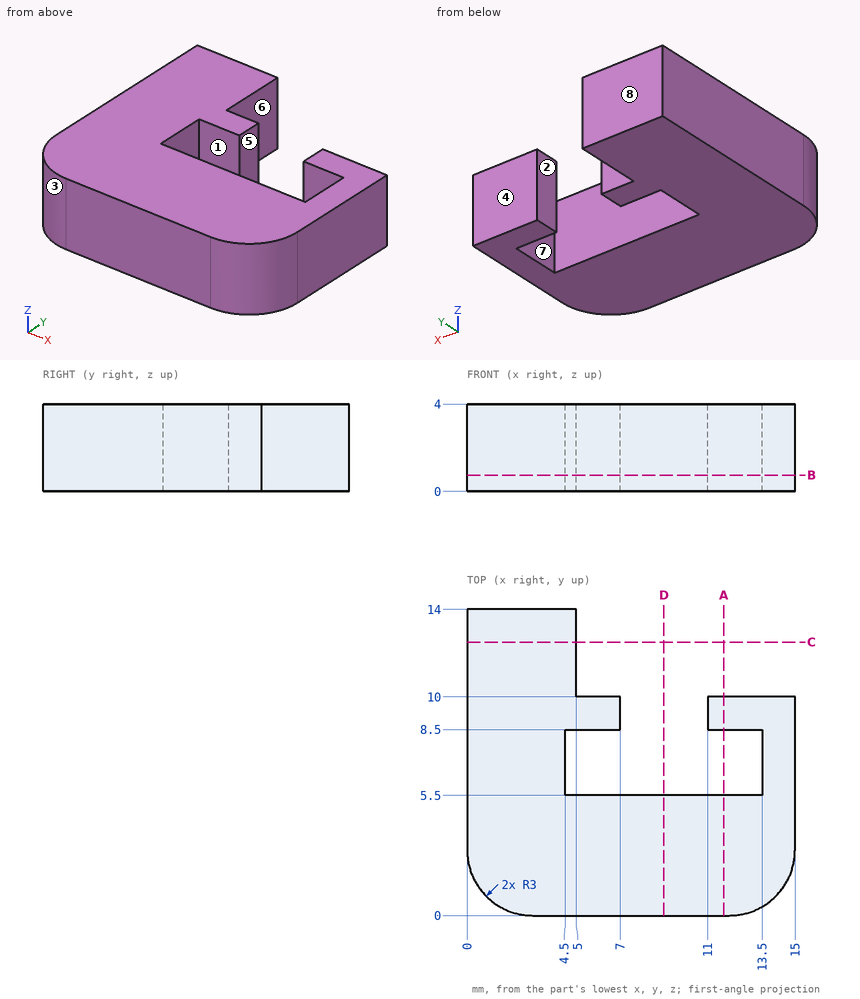
For this review, use the dimensioned drawing (mm, ordinates from the lowest corner) and the shaded views. A direction names the side the tool comes from. Give positions to 0.01 mm unless a question says otherwise; leave off trailing zeros. Order: outer loops, then holes, each group sorted by start corner. A loop starts at its lowest first (then second) coordinate and runs counter-clockwise, first axis right, second up.
1. Add section A-A, the plane x = 11.75. State the section outline as (y, z) points.
Solution:
outline: (0, 0) - (5.5, 0) - (5.5, 4) - (0, 4) - close; (8.5, 0) - (10, 0) - (10, 4) - (8.5, 4) - close
2. To check wall thickness, follow L1, parallel to X at y = 9.5, z = 0.5; L2, parallel to Y at x = 6, z = 2.2; L3, parallel to X at y = 7, z = 2.3. State the ranges of each line that lie inside material, in increasing order.
Solution:
L1: x = 0 to 7, 11 to 15
L2: y = 0 to 5.5, 8.5 to 10
L3: x = 0 to 4.5, 13.5 to 15
3. Add section C-C, the plane y = 12.5. State the section outline as (x, z) points, then the cut area to 3 significant figures.
Solution:
outline: (0, 0) - (5, 0) - (5, 4) - (0, 4) - close
area: 20.0 mm2
4. Add section B-B, the plane z = 0.75. State the section outline as (x, y) points, then the cut area to 3 significant figures.
Solution:
outline: (0, 3) arc R3 ccw to (3, 0) - (12, 0) arc R3 ccw to (15, 3) - (15, 10) - (11, 10) - (11, 8.5) - (13.5, 8.5) - (13.5, 5.5) - (4.5, 5.5) - (4.5, 8.5) - (7, 8.5) - (7, 10) - (5, 10) - (5, 14) - (0, 14) - close
area: 133 mm2
5. Tool access review of the marked faces 1, 2, 3 and 4: name each direction out of +Z, -Z, +X, -X, +Y, -Y from which nothing blocks a thin tool from reaching the whole face with its end or side.
Solution:
face 1: +Z, -Z
face 2: +Z, -Z, +Y
face 3: +Z, -Z, -X, -Y
face 4: +Z, -Z, +X, +Y
6. Mouldability with a two-part tool opening along X and no side actions: class the marked faces 5, 6, 7 and 8 as +X half, -X half, draft (parallel to the pull), parting line (faces both ways), or undercut.
Solution:
face 5: undercut
face 6: +X half
face 7: undercut
face 8: draft
7. Add section D-D, the plane x = 9. State the section outline as (y, z) points.
Solution:
outline: (0, 0) - (5.5, 0) - (5.5, 4) - (0, 4) - close
8. For pin 1 Ø2 at (x, z) = (13.5, 1.5) entering from +Y; pin 2 Ø5 at (x, y) = (3.5, 11.5) entering from -Z, all flat-tipped, find the tip position at first contact; note any pin that passes through.
Solution:
pin 1: stops at y = 10
pin 2: stops at z = 0
